```python
from build123d import *

# Parameters (mm, degrees)
SKETCH1_W           = 80
SKETCH1_H           = 30
BOSS_EXTRUDE1_DEPTH = 3
SKETCH2_R           = 1.5
SKETCH2_R_2         = 2
CUT_EXTRUDE2_DEPTH  = 4


with BuildPart() as part:
    # Sketch1 → Boss-Extrude1 (new body)
    with BuildSketch(Plane.XY):
        Rectangle(SKETCH1_W, SKETCH1_H)
    extrude(amount=BOSS_EXTRUDE1_DEPTH)

    # Sketch2 → Cut-Extrude2 (cut, through all)
    with BuildSketch(Plane.XY.offset(3)):
        with Locations((37, 12)):
            Circle(SKETCH2_R)
        with Locations((-37, 12)):
            Circle(SKETCH2_R)
        with Locations((37, -12)):
            Circle(SKETCH2_R)
        with Locations((-37, -12)):
            Circle(SKETCH2_R)
        with Locations((-14, 0)):
            Circle(SKETCH2_R_2)
        with Locations((-34, 0)):
            Circle(SKETCH2_R_2)
        with Locations((16.33, 0)):
            Circle(SKETCH2_R_2)
        with BuildLine():
            Line((-34.032472505, 12.440205142), (-15.8, 12.440205142))
            Line((-15.8, 12.440205142), (-15.8, 3.57211422))
            ThreePointArc((-15.8, 3.57211422), (-16.489437492, 3.130926536), (-17.074634359, 2.558637051))
            Line((-17.074634359, 2.558637051), (-30.925365641, 2.558637051))
            ThreePointArc((-30.925365641, 2.558637051), (-32.306522762, 3.623828755), (-34.009676412, 3.999988296))
            Line((-34.009676412, 3.999988296), (-34.009676412, 11.759241116))
            ThreePointArc((-34.009676412, 11.759241116), (-34.001679573, 12.100372396), (-34.032472505, 12.440205142))
        make_face()
        with BuildLine():
            Line((13.32333178, 2.638170998), (-10.99333178, 2.638170998))
            ThreePointArc((-10.99333178, 2.638170998), (-11.595928807, 3.196942555), (-12.3, 3.620773398))
            Line((-12.3, 3.620773398), (-12.3, 12))
            Line((-12.3, 12), (14.63, 12))
            Line((14.63, 12), (14.63, 3.620773398))
            ThreePointArc((14.63, 3.620773398), (13.925928807, 3.196942555), (13.32333178, 2.638170998))
        make_face()
        with BuildLine():
            Line((35, 2.571779372), (19.393649925, 2.571779372))
            ThreePointArc((19.393649925, 2.571779372), (18.812728358, 3.136249336), (18.13, 3.57211422))
            Line((18.13, 3.57211422), (18.13, 12))
            Line((18.13, 12), (34, 12))
            ThreePointArc((34, 12), (34.261387212, 10.775255129), (35, 9.763932023))
            Line((35, 9.763932023), (35, 2.571779372))
        make_face()
    cut_extrude2 = extrude(amount=-CUT_EXTRUDE2_DEPTH, mode=Mode.SUBTRACT)

    # Mirror1: Cut-Extrude2 across plane
    add(cut_extrude2.mirror(Plane.ZX), mode=Mode.SUBTRACT)


solid = part.part
```
Here's how the part is built. I have some questions about the finished solid (model axes, mm). Coordinates: 2 decimals unless noted, no trailing zeros. Order: outer loops, then holes, each group sorted by start corner. A loop starts at its lowest first (then second) coordinate and runs counter-clockwise, first axis right, second up. Notation, with made-up numbers: (10.5, 5.5) - (52.5, 5.5) arc R30 ccw to (52.5, 37.5) - close; hole circle Ø8 at (32, 33.25). An arc over 180 degrees is marked (long way). One line per question, with ' | ' between items.
(1) Will this pin go through, and if not, where does the flat tip stop? pin 1 (2.5 mm diameter, centred on x = -37, y = -12, fed in from -Z).
Report:
pin 1: passes through
(2) If I drill on L1, parallel to Y at x = -9.5, z = 1; L2, parallel to X at y = 4.5, z = 2; L3, parallel to Y at x = -29, z = 2.2, over which ranges is the centre line in solid material (lowest first)?
Report:
L1: y = -15 to -12, -2.64 to 2.64, 12 to 15 | L2: x = -40 to -34.01, -15.8 to -12.3, 14.63 to 18.13, 35 to 40 | L3: y = -15 to -12.44, -2.56 to 2.56, 12.44 to 15
(3) Suppose I cut it at A-A on x = 37. List the corners of the cut face in (y, z) for me, and give its area (3 significant figures).
Report:
outline: (-15, 0) - (-13.5, 0) - (-13.5, 3) - (-15, 3) - close; (-10.5, 0) - (10.5, 0) - (10.5, 3) - (-10.5, 3) - close; (13.5, 0) - (15, 0) - (15, 3) - (13.5, 3) - close | area: 72.0 mm2
(4) Suppose I cut it at C-C on y = -8.25. List the corners of the cut face in (x, z) for me, and give its area (3 significant figures).
Report:
outline: (-40, 0) - (-34.01, 0) - (-34.01, 3) - (-40, 3) - close; (-15.8, 0) - (-12.3, 0) - (-12.3, 3) - (-15.8, 3) - close; (14.63, 0) - (18.13, 0) - (18.13, 3) - (14.63, 3) - close; (35, 0) - (40, 0) - (40, 3) - (35, 3) - close | area: 54.0 mm2
(5) Suppose I cut it at B-B on x = -14. List the corners of the cut face in (y, z) for me, and give its area (3 significant figures).
Report:
outline: (-15, 0) - (-2, 0) - (-2, 3) - (-15, 3) - close; (2, 0) - (15, 0) - (15, 3) - (2, 3) - close | area: 78.0 mm2
(6) Suppose I cut it at D-D on z = 0.7. State how many separate pieces and enclosed holes the cut face has, and give its area (3 significant figures).
Report:
separate pieces: 1 | enclosed holes: 13 | area: 1,170 mm2
